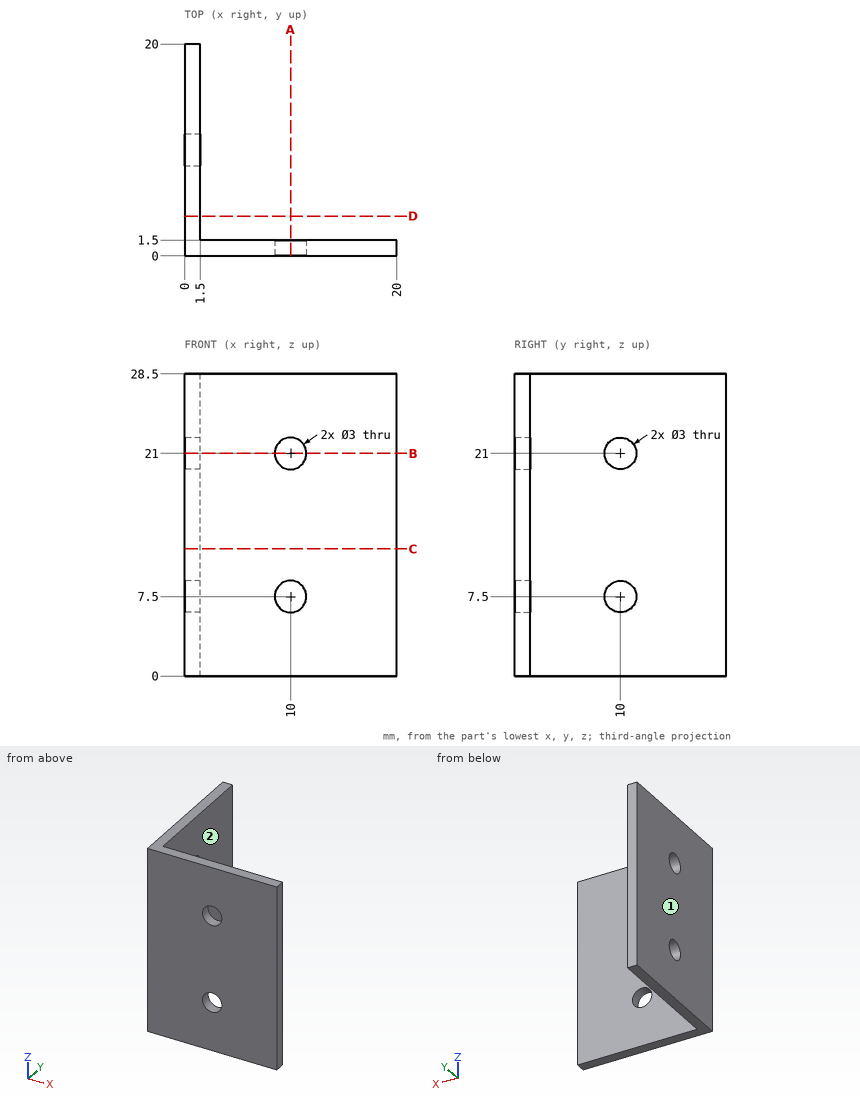
Verification items for this drawing (mm, ordinates from the low corner). A direction names the side the tool comes from. Coordinates: 2 decimals unless noted, no trailing zeros. Order: outer loops, then holes, each group sorted by start corner. A loop starts at its lowest first (then second) coordinate and runs counter-clockwise, first axis right, second up. Notation, with made-up numbers: M -21.75,38 L -16.75,38 A33 ccw -16.75,67 Z; hole C -22,38 d7. An arc over 180 degrees is marked long. One line per item, written item: value. Start each with the question number.
Item 1: Sectioned sample at C-C on z = 12. Record the cut outline in (x, y).
Item 2: Sectioned sample at A-A on x = 10. Record the cut outline in (y, z).
Item 3: Access from +Z, -Z, +X, -X, +Y, -Y to the whole of each face (thin tool, end or side, straight path). Record for the marked faces 1 and 2.
Item 4: Sectioned sample at D-D on y = 3.75. Record the cut outline in (x, z), then the cut area to 4 significant figures.
Item 5: Thickness scan on probe 1 along Z at (x, y) = (0.55, 10); probe 2 along X at (y, z) = (0.7, 7.5); probe 3 along Y at (x, z) = (7.25, 25.25). Record the ranges inside material, lowest first.
Item 6: Depth check by flat-ended pin: P1, Ø2.5, axis at x = 10, z = 21, coming from the +Y side; P2, Ø8, axis at y = 14, z = 20, coming from the +X side; P3, Ø1.5, axis at x = 6.5, z = 13, coming from the +Y side. Enter the tip coordinate at first touch or a pass-through.
Item 7: Sectioned sample at B-B on z = 21. Record the cut outline in (x, y).
Calculated:
1. outline: M 0,0 L 20,0 L 20,1.5 L 1.5,1.5 L 1.5,20 L 0,20 Z
2. outline: M 0,0 L 1.5,0 L 1.5,6 L 0,6 Z; M 0,9 L 1.5,9 L 1.5,19.5 L 0,19.5 Z; M 0,22.5 L 1.5,22.5 L 1.5,28.5 L 0,28.5 Z
3. face 1: +Z, -Z, -X, +Y, -Y
3. face 2: +Z, -Z, +X, +Y
4. outline: M 0,0 L 1.5,0 L 1.5,28.5 L 0,28.5 Z
4. area: 42.75 mm^2
5. probe 1: 0 to 6, 9 to 19.5, 22.5 to 28.5
5. probe 2: 0 to 8.5, 11.5 to 20
5. probe 3: 0 to 1.5
6. P1: through
6. P2: x = 1.5
6. P3: y = 1.5
7. outline: M 0,0 L 8.5,0 L 8.5,1.5 L 1.5,1.5 L 1.5,8.5 L 0,8.5 Z; M 0,11.5 L 1.5,11.5 L 1.5,20 L 0,20 Z; M 11.5,0 L 20,0 L 20,1.5 L 11.5,1.5 Z
